Read the model definition and answer for the solid it produces. Units are mm, in the model's axes. Face numbers are marked on the shaded views. A direction names the side the tool comes from. Round coordinates to 2 decimals unless told otherwise and drop trailing zeros. Order: outer loops, then holes, each group sorted by start corner. A loop starts at its lowest first (then second) coordinate and runs counter-clockwise, first axis right, second up.
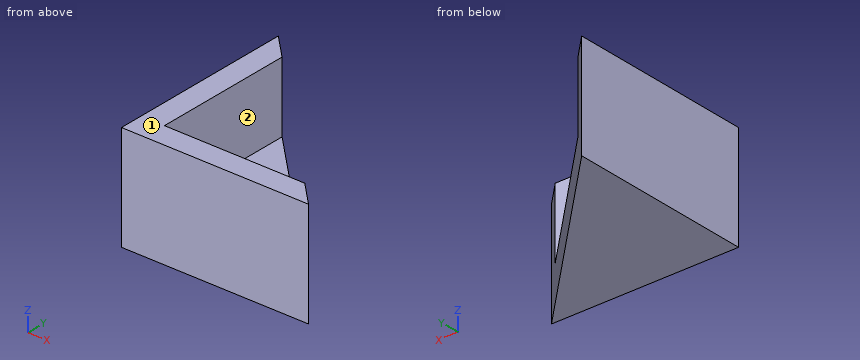
from build123d import *

# Parameters (mm, degrees)
F1_DEPTH = 1.5
F3_DEPTH = 3


with BuildPart() as f1:
    # F0 (on Top) → F1 (new body)
    with BuildSketch(Plane.XY):
        Polygon((0, 8), (0, 0), (8, 0), align=None)
    extrude(amount=F1_DEPTH)

    # F2 (on face) → F3 (join)
    with BuildSketch(Plane.XY.offset(1.5)):
        Polygon((1, 1), (1, 7), (0, 8), (0, 0), (8, 0), (7, 1), align=None)
    extrude(amount=F3_DEPTH)


solid = f1.part
Q1. A cutting plane is placed at B-B, the plane x = 3. Give the vertices of the cut face in (y, z), plus the area to 3 significant figures.
Outcome:
outline: (0, 0) - (5, 0) - (5, 1.5) - (1, 1.5) - (1, 4.5) - (0, 4.5) - close
area: 10.5 mm2
Q2. Straight lines are drawn through the part: probe 1 along X at (y, z) = (1.75, 3.85); probe 2 along Z at (x, y) = (1.5, 3.25). For each, find the intervals that lie inside material, in ascending order.
Outcome:
probe 1: x = 0 to 1
probe 2: z = 0 to 1.5
Q3. Flat-ended cylindrical pins translate along their axes: pin 1 (1 mm diameter, centred on x = 5, z = 3.5, fed in from +Y); pin 2 (1.8 mm diameter, centred on x = 3.5, y = 4.5, fed in from +Z); pin 3 (1.5 mm diameter, centred on y = 2.5, z = 3, fed in from +X). Find the tip coordinate at first contact, or state that the pin passes through.
Outcome:
pin 1: stops at y = 1
pin 2: stops at z = 1.5
pin 3: stops at x = 1
Q4. A cutting plane is placed at D-D, the plane y = 0.5. Give the vertices of the cut face in (x, z), plus the area to 4 significant figures.
Outcome:
outline: (0, 0) - (7.5, 0) - (7.5, 4.5) - (0, 4.5) - close
area: 33.75 mm2
Q5. A cutting plane is placed at A-A, the plane y = 5.5. Give the vertices of the cut face in (x, z).
Outcome:
outline: (0, 0) - (2.5, 0) - (2.5, 1.5) - (1, 1.5) - (1, 4.5) - (0, 4.5) - close
Q6. A cutting plane is placed at C-C, the plane z = 0.55. Give the vertices of the cut face in (x, y), plus the area to 3 significant figures.
Outcome:
outline: (0, 0) - (8, 0) - (0, 8) - close
area: 32.0 mm2
Q7. For the marked faces 1 and 2, determine the directions among +Z, -Z, +X, -X, +Y, -Y from which every point of the face is accessible in a straight line to the end or side of a thin tool.
Outcome:
face 1: +Z, +X, -X, +Y, -Y
face 2: +Z, +X, +Y
